Input: part model. Units: mm. Frame: model coordinates. A direction names the side the tool comes from. Coordinates: 2 decimals unless noted, no trailing zeros. Loops run counter-clockwise (first coordinate to the right, second up) from the corner with the lowest first, then second, coordinate; pieces in that order, holes last. Notation, with made-up numbers: (32, 44) - (75, 44) arc R21 cw to (75, 68) - close; hole circle Ø1 at (4.5, 70.25). An arc over 180 degrees is marked (long way). Use a Markdown table: item, result. Add a question column.
1. Section query B-B on x = 0. Return the cut outline in (y, z).
2. Section query A-A on y = 10.16. Return the cut outline in (x, z).
3. Draft query along X for faces 3 (the face through (3, 13, 12.7)), 4 (the face through (3.778, 2.504, -0.496)), 5 (the face through (12.7, 4, 6)). Return one class per face: released by +X, released by -X, zero draft, split by the parting line, or undercut.
4. Ray query, L1, parallel to Y at x = 0, z = 11.35; L2, parallel to Z at x = 4.5, y = 15; L3, parallel to Y at x = 1.25, z = 7.75. Return the intervals inside material, ascending. Write a range as [from, to].
5. Section query D-D on x = 7.25. Return the cut outline in (y, z).
6. Section query C-C on z = 0. Return the cut outline in (x, y).
7. Access query for faces 1 (the face through (0, 15, 7.62)), 2 (the face through (-1.172, 18.067, 10.124)). Directions: +Z, -Z, +X, -X, +Y, -Y. A direction counts if a zero-diameter tool reaches every point of the face in a straight line with its end or side. Return the directions, or none.
8. Contact query for flat-ended pins moving along their axis: P1, Ø12, axis at x = 1, y = 8, coming from the +Z side; P2, Ø10, axis at x = 2, y = 16, coming from the -Z side; P3, Ø9, axis at x = 0, z = 0, coming from the +Y side; P4, Ø4.5, axis at x = 0, y = 10.16, coming from the -Z side. Output: stop coordinate, or through.
```python
from build123d import *

# Parameters (mm, degrees)
SKETCH2_W           = 25.4
SKETCH2_H           = 25.4
SKETCH2_R           = 3.81
BOSS_EXTRUDE1_DEPTH = 5.08
SKETCH3_W           = 25.4
SKETCH3_H           = 5.08
BOSS_EXTRUDE2_DEPTH = 20.32
SKETCH4_R           = 2.54
CUT_EXTRUDE1_DEPTH  = 35.919226796


with BuildPart() as part:
    # Sketch2 → Boss-Extrude1 (new body)
    with BuildSketch(Plane(origin=(0, 0, 0), x_dir=(1, 0, 0), z_dir=(0, 1, 0))):
        Rectangle(SKETCH2_W, SKETCH2_H)
        with Locations(Location((0, 0, 0), (0, 0, 270))):
            Circle(SKETCH2_R, mode=Mode.SUBTRACT)
    extrude(amount=BOSS_EXTRUDE1_DEPTH)

    # Sketch3 → Boss-Extrude2 (add)
    with BuildSketch(Plane(origin=(0, 5.08, 0), x_dir=(1, 0, 0), z_dir=(0, 1, 0))):
        with Locations((0, -10.16)):
            Rectangle(SKETCH3_W, SKETCH3_H)
    extrude(amount=BOSS_EXTRUDE2_DEPTH)

    # Sketch4 → Cut-Extrude1 (cut, through all)
    with BuildSketch(Plane(origin=(0, 0, 7.62), x_dir=(-1, 0, 0), z_dir=(0, 0, -1))):
        with Locations((0, 20.32)):
            Circle(SKETCH4_R)
        with Locations((0, 10.16)):
            Circle(SKETCH4_R)
    extrude(amount=-CUT_EXTRUDE1_DEPTH, mode=Mode.SUBTRACT)


solid = part.part
```
Resolved:
| question | item | result |
|---|---|---|
| 1 | outline | (0, -12.7) - (5.08, -12.7) - (5.08, -3.81) - (0, -3.81) - close; (0, 3.81) - (5.08, 3.81) - (5.08, 7.62) - (7.62, 7.62) - (7.62, 12.7) - (0, 12.7) - close; (12.7, 7.62) - (17.78, 7.62) - (17.78, 12.7) - (12.7, 12.7) - close; (22.86, 7.62) - (25.4, 7.62) - (25.4, 12.7) - (22.86, 12.7) - close |
| 2 | outline | (-12.7, 7.62) - (-2.54, 7.62) - (-2.54, 12.7) - (-12.7, 12.7) - close; (2.54, 7.62) - (12.7, 7.62) - (12.7, 12.7) - (2.54, 12.7) - close |
| 3 | face 3 | zero draft |
| 3 | face 4 | undercut |
| 3 | face 5 | released by +X |
| 4 | L1 | [0, 7.62], [12.7, 17.78], [22.86, 25.4] |
| 4 | L2 | [7.62, 12.7] |
| 4 | L3 | [0, 7.95], [12.37, 18.11], [22.53, 25.4] |
| 5 | outline | (0, -12.7) - (5.08, -12.7) - (5.08, 7.62) - (25.4, 7.62) - (25.4, 12.7) - (0, 12.7) - close |
| 6 | outline | (-12.7, 0) - (-3.81, 0) - (-3.81, 5.08) - (-12.7, 5.08) - close; (3.81, 0) - (12.7, 0) - (12.7, 5.08) - (3.81, 5.08) - close |
| 7 | face 1 | -Z, +X, -X, +Y |
| 7 | face 2 | +Z, -Z |
| 8 | P1 | z = 12.7 |
| 8 | P2 | z = 7.62 |
| 8 | P3 | y = 5.08 |
| 8 | P4 | through |
